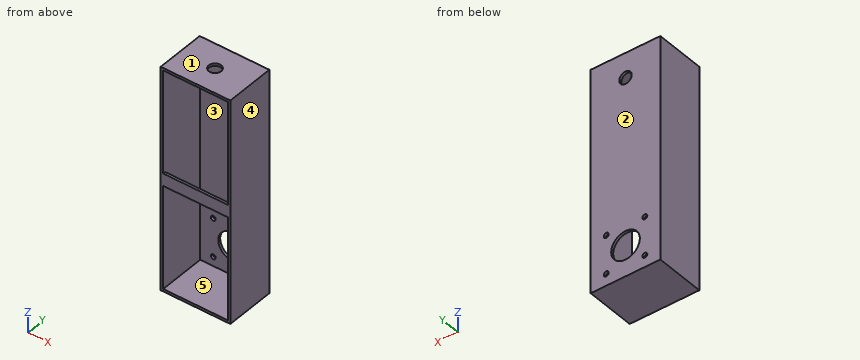
Autodesk Inventor part; units mm, degrees
ref_plane "YZ Plane" through (0, 0, 0) normal (1, 0, 0) x (0, 1, 0)
ref_plane "XZ Plane" through (0, 0, 0) normal (0, 1, 0) x (-1, 0, 0)
ref_plane "XY Plane" through (0, 0, 0) normal (0, 0, 1) x (1, 0, 0)
sketch "Sketch1" plane through (0, 0, 0) normal (0, 0, 1) x (1, 0, 0)
  line L0 (-28, 0) -> (28, 0)
  line L1 (28, 0) -> (28, 40)
  line L2 (28, 40) -> (-28, 40)
  line L3 (-28, 40) -> (-28, 0)
  point P0 (0, 0)
  point P1 (0, 0)
  dimension "d1" = 56
  dimension "d2" = 40
extrude "Extrusion1" add sketch "Sketch1" along normal mid plane 180
shell "Shell1" thickness 2 removed faces 1 at (-9.3333, 0, 30)
sketch "Sketch2" plane through (0, 0, 90) normal (0, 0, 1) x (1, 0, 0)
  circle A0 centre (0, 20) radius 5
  line L0 (-28, 0) -> (28, 0) construction
  line L1 (28, 0) -> (28, 40) construction
  point P0 (0, 0)
  point P1 (0, 0)
  point P2 (28, 20)
  dimension "d6" = 10
extrude "Extrusion2" cut sketch "Sketch2" against normal up to surface (2 mm away)
sketch "Sketch3" plane through (-28, 40, 90) normal (0, 1, 0) x (1, 0, 0)
  line L0 (56, 180) -> (56, 0) construction
  line L1 (56, 40) -> (0, 40) construction
  circle A0 centre (28, 155) radius 11.5
  circle A1 centre (12.5, 139.5) radius 2
  circle A2 centre (43.5, 170.5) radius 2
  circle A3 centre (12.5, 170.5) radius 2
  circle A4 centre (43.5, 139.5) radius 2
  line L2 (43.5, 139.5) -> (12.5, 139.5) construction
  line L3 (12.5, 139.5) -> (12.5, 170.5) construction
  line L4 (12.5, 170.5) -> (43.5, 170.5) construction
  line L5 (43.5, 170.5) -> (43.5, 139.5) construction
  line L6 (43.5, 139.5) -> (12.5, 170.5) construction
  line L7 (0, 0) -> (56, 0) construction
  line L8 (56, 0) -> (0, 40) construction
  line L9 (0, 180) -> (0, 0) construction
  circle A5 centre (28, 20) radius 5
  point P0 (28, 90)
  dimension "d9" = 40
  dimension "d10" = 4
  dimension "d11" = 23
  dimension "d12" = 115
  dimension "d13" = 31
  dimension "d16" = 10
extrude "Extrusion3" cut sketch "Sketch3" against normal up to surface (2 mm away)
sketch "Sketch4" plane through (-28, 0, 90) normal (0, -1, 0) x (1, 0, 0)
  line L0 (2, -178) -> (2, -2)
  line L1 (54, -95) -> (2, -95)
  line L2 (2, -95) -> (2, -85)
  line L3 (2, -85) -> (54, -85)
  line L4 (54, -85) -> (54, -95)
  line L5 (54, -95) -> (2, -85) construction
  line L6 (2, -95) -> (54, -85) construction
  point P0 (28, -90)
  dimension "d17" = 10
extrude "Extrusion4" add sketch "Sketch4" against normal blind 2
properties part number "Soporte_base"
Source: CAD feature listing. Evaluate the final solid. Frame: model axes, mm. Face numbers are marked on the shaded views. A direction names the side the tool comes from. Coordinates: 2 decimals unless noted, no trailing zeros. Loops run counter-clockwise (first coordinate to the right, second up) from the corner with the lowest first, then second, coordinate; pieces in that order, holes last. Notation, with made-up numbers: (33.5, 68) - (75.5, 68) arc R29 ccw to (75.5, 89) - close; hole circle Ø8 at (-37, -0.75). An arc over 180 degrees is marked (long way). One line per item, written item: value. Start each with the question number.
1. Section A-A (z = -49.5). Return the cut outline in (x, y), and give its area (3 significant figures).
2. Ray query, L1, parallel to X at y = 38.75, z = -80.5; L2, parallel to Z at x = 15.5, y = 38.5; L3, parallel to Z at x = 0, y = 38.55. Return the intervals inside material, ascending.
3. Section D-D (x = -15.5). Return the cut outline in (y, z).
4. Mould query, pull axis Z, two halves, no side actions, for the marked faces 1, 2 and 3. Classes: pulls with the +Z half, pulls with the -Z half, needs draft (parallel to the pull), parting line crosses it, or undercut.
5. Set-up query: the marked faces 4 and 5. Return all of +Z, -Z, +X, -X, +Y, -Y with unobstructed straight access to the full face (end or side cutting, diameter ignored); none if empty.
6. Contact query for flat-ended pins moving along their axis: P1, Ø10, axis at x = 13.5, z = 29, coming from the -Y side; P2, Ø20.5, axis at x = 0, z = -65, coming from the -Y side; P3, Ø4.5, axis at x = 15.5, z = -49.5, coming from the +Y side. Output: stop coordinate, or through.
7. Section B-B (x = 0). Return the cut outline in (y, z), and give its area (3 significant figures).
8. Section C-C (y = 9). Return the cut outline in (x, z).
Verdict:
1. outline: (-28, 0) - (-26, 0) - (-26, 38) - (-17.5, 38) - (-17.5, 40) - (-28, 40) - close; (-13.5, 38) - (13.5, 38) - (13.5, 40) - (-13.5, 40) - close; (17.5, 38) - (26, 38) - (26, 0) - (28, 0) - (28, 40) - (17.5, 40) - close
1. area: 248 mm2
2. L1: x = -28 to -17.5, -13.5 to 13.5, 17.5 to 28
2. L2: z = -90 to -82.5, -78.5 to -51.5, -47.5 to 90
2. L3: z = -90 to -76.5, -53.5 to 65, 75 to 90
3. outline: (0, -90) - (40, -90) - (40, -82.5) - (38, -82.5) - (38, -88) - (0, -88) - close; (0, -5) - (2, -5) - (2, 5) - (0, 5) - close; (0, 88) - (38, 88) - (38, -47.5) - (40, -47.5) - (40, 90) - (0, 90) - close; (38, -78.5) - (40, -78.5) - (40, -51.5) - (38, -51.5) - close
4. face 1: pulls with the +Z half
4. face 2: needs draft
4. face 3: undercut
5. face 4: +Z, -Z, +X, +Y, -Y
5. face 5: -Y
6. P1: stops at y = 38
6. P2: passes through
6. P3: stops at y = 40
7. outline: (0, -90) - (40, -90) - (40, -76.5) - (38, -76.5) - (38, -88) - (0, -88) - close; (0, -5) - (2, -5) - (2, 5) - (0, 5) - close; (0, 88) - (15, 88) - (15, 90) - (0, 90) - close; (25, 88) - (38, 88) - (38, 75) - (40, 75) - (40, 90) - (25, 90) - close; (38, -53.5) - (40, -53.5) - (40, 65) - (38, 65) - close
7. area: 446 mm2
8. outline: (-28, -90) - (28, -90) - (28, 90) - (-28, 90) - close; hole (-26, -88) - (26, -88) - (26, 88) - (-26, 88) - close
